```python
from build123d import *

# Parameters (mm, degrees)
SKETCH1_R     = 1
BODY_DEPTH    = 1.2
FILLET1_R     = 0.5
FILLET2_R     = 1
SCALE_1_SCALE = 0.25


with BuildPart() as part:
    # Sketch1 → Body (new body)
    with BuildSketch(Plane.XY):
        with BuildLine():
            Line((-1.25, -11.859392549), (-1.25, -16.279514555))
            ThreePointArc((-1.25, -16.279514555), (-4.178435105, -15.756174328), (-6.952957407, -14.683027947))
            Line((-6.952957407, -14.683027947), (-7.547042593, -11.313803432))
            ThreePointArc((-7.547042593, -11.313803432), (0, 13.6), (7.547042593, -11.313803432))
            Line((7.547042593, -11.313803432), (6.952957407, -14.683027947))
            ThreePointArc((6.952957407, -14.683027947), (4.178435105, -15.756174328), (1.25, -16.279514555))
            Line((1.25, -16.279514555), (1.25, -11.859392549))
            ThreePointArc((1.25, -11.859392549), (0, 10.27), (-1.25, -11.859392549))
        make_face()
        with Locations(Location((4.25, -13.432678287, 0), (0, 0, 180))):
            Circle(SKETCH1_R, mode=Mode.SUBTRACT)
        with Locations((-4.25, -13.432678287)):
            Circle(SKETCH1_R, mode=Mode.SUBTRACT)
    extrude(amount=-BODY_DEPTH)

    # Fillet1
    fillet1_edges = [part.edges().sort_by_distance(p)[0] for p in [
        (-6.952957407, -14.683027947, -0.6),
        (6.952957407, -14.683027947, -0.6),
    ]]
    fillet(fillet1_edges, radius=FILLET1_R)

    # Fillet2
    fillet2_edges = [part.edges().sort_by_distance(p)[0] for p in [
        (-7.547042593, -11.313803432, -0.6),
        (7.547042593, -11.313803432, -0.6),
    ]]
    fillet(fillet2_edges, radius=FILLET2_R)


with BuildPart() as part_1:
    # 缩放比例1: scaled about (0, 0, 0)
    add(part.part.scale(SCALE_1_SCALE))


solid = part_1.part
```
Here's how the part is built. I have some questions about the finished solid (model axes, mm). Give positions to 0.01 mm unless a question says otherwise; leave off trailing zeros. Order: outer loops, then holes, each group sorted by start corner. A loop starts at its lowest first (then second) coordinate and runs counter-clockwise, first axis right, second up. Notation, with made-up numbers: (-11.75, 1) -> (41.25, 1) arc R11 ccw to (41.25, 12) -> close; hole circle Ø5 at (-31, -5.75). An arc over 180 degrees is marked (long way). Use CSV: the item, a comma, the result in double quotes. Start each with the question number.
Item 1: Suppose I cut it at D-D (y = -3.5). List the corners of the cut face in (x, z) for me.
Item 2: If I drill on probe 1 along X at (y, z) = (1.5, -0.15); probe 2 along X at (y, z) = (2.25, -0.05); probe 3 along Y at (x, z) = (-2, -0.2), over which ranges is the centre line in solid material (lowest first)? Write a range as [from, to].
Item 3: Suppose I cut it at B-B (x = -0.5). List the corners of the cut face in (y, z) for me.
Item 4: Suppose I cut it at C-C (z = -0.1). Give the number of separate pieces and of enclosed holes in the cut face, and give its area (3 significant figures).
Item 5: Suppose I cut it at A-A (y = 1.5). List the corners of the cut face in (x, z) for me, and give its area (3 significant figures).
Answer block:
1,outline,"(-1.77, -0.3) -> (-1.27, -0.3) -> (-1.27, 0) -> (-1.77, 0) -> close; (-0.86, -0.3) -> (-0.31, -0.3) -> (-0.31, 0) -> (-0.86, 0) -> close; (0.31, -0.3) -> (0.86, -0.3) -> (0.86, 0) -> (0.31, 0) -> close; (1.27, -0.3) -> (1.77, -0.3) -> (1.77, 0) -> (1.27, 0) -> close"
2,probe 1,"x = [-3.05, -2.19], [2.19, 3.05]"
2,probe 2,"x = [-2.55, -1.29], [1.29, 2.55]"
2,probe 3,"y = [-2.75, -2.13], [1.72, 2.75]"
3,outline,"(-4.05, -0.3) -> (-2.94, -0.3) -> (-2.94, 0) -> (-4.05, 0) -> close; (2.52, -0.3) -> (3.36, -0.3) -> (3.36, 0) -> (2.52, 0) -> close"
4,separate pieces,"1"
4,enclosed holes,"2"
4,area,"13.6 mm^2"
5,outline,"(-3.05, -0.3) -> (-2.19, -0.3) -> (-2.19, 0) -> (-3.05, 0) -> close; (2.19, -0.3) -> (3.05, -0.3) -> (3.05, 0) -> (2.19, 0) -> close"
5,area,"0.518 mm^2"
